Read the model definition and answer for the solid it produces. Units are mm, in the model's axes. Face numbers are marked on the shaded views. A direction names the side the tool comes from. Coordinates: 2 decimals unless noted, no trailing zeros. Order: outer loops, then holes, each group sorted by start corner. A loop starts at its lowest first (then second) coordinate and runs counter-clockwise, first axis right, second up.
from build123d import *

# Parameters (mm, degrees)
SZKIC1_W                    = 57.14
SZKIC1_H                    = 57.14
SZKIC1_R                    = 2.5
DODANIE_WYCI_GNI_CIE1_DEPTH = 5
DODANIE_WYCI_GNI_CIE2_DEPTH = 71
ZAOKR_GLENIE1_R             = 2
SZKIC3_R                    = 4
DODANIE_WYCI_GNI_CIE3_DEPTH = 20.6
ZAOKR_GLENIE2_R             = 5


with BuildPart() as part:
    # Szkic1 → Dodanie-wyciągnięcie1 (new body)
    with BuildSketch(Plane(origin=(0, 0, 0), x_dir=(1, 0, 0), z_dir=(0, 1, 0))):
        Rectangle(SZKIC1_W, SZKIC1_H)
        with Locations(Location((-23.57, 23.57, 0), (0, 0, 270))):
            Circle(SZKIC1_R, mode=Mode.SUBTRACT)
        with Locations(Location((23.57, 23.57, 0), (0, 0, 270))):
            Circle(SZKIC1_R, mode=Mode.SUBTRACT)
        with Locations(Location((23.57, -23.57, 0), (0, 0, 270))):
            Circle(SZKIC1_R, mode=Mode.SUBTRACT)
        with Locations(Location((-23.57, -23.57, 0), (0, 0, 270))):
            Circle(SZKIC1_R, mode=Mode.SUBTRACT)
    extrude(amount=DODANIE_WYCI_GNI_CIE1_DEPTH)

    # Szkic2 → Dodanie-wyciągnięcie2 (add)
    with BuildSketch(Plane(origin=(0, 5, 0), x_dir=(1, 0, 0), z_dir=(0, 1, 0))):
        with BuildLine():
            ThreePointArc((-19.07, 23.57), (-20.388019485, 20.388019485), (-23.57, 19.07))
            Line((-23.57, 19.07), (-28.57, 19.07))
            Line((-28.57, 19.07), (-28.57, -19.07))
            Line((-28.57, -19.07), (-23.57, -19.07))
            ThreePointArc((-23.57, -19.07), (-20.388019485, -20.388019485), (-19.07, -23.57))
            Line((-19.07, -23.57), (-19.07, -28.57))
            Line((-19.07, -28.57), (19.07, -28.57))
            Line((19.07, -28.57), (19.07, -23.57))
            ThreePointArc((19.07, -23.57), (20.388019485, -20.388019485), (23.57, -19.07))
            Line((23.57, -19.07), (28.57, -19.07))
            Line((28.57, -19.07), (28.57, 19.07))
            Line((28.57, 19.07), (23.57, 19.07))
            ThreePointArc((23.57, 19.07), (20.388019485, 20.388019485), (19.07, 23.57))
            Line((19.07, 23.57), (19.07, 28.57))
            Line((19.07, 28.57), (-19.07, 28.57))
            Line((-19.07, 28.57), (-19.07, 23.57))
        make_face()
    extrude(amount=DODANIE_WYCI_GNI_CIE2_DEPTH)

    # Zaokrąglenie1
    zaokr_glenie1_edges = [part.edges().sort_by_distance(p)[0] for p in [
        (19.07, 76, 26.07),
        (0, 76, 28.57),
        (-19.07, 76, 26.07),
        (-20.388019485, 76, 20.388019485),
        (-26.07, 76, 19.07),
        (-28.57, 76, 0),
        (-26.07, 76, -19.07),
        (-20.388019485, 76, -20.388019485),
        (-19.07, 76, -26.07),
        (0, 76, -28.57),
        (19.07, 76, -26.07),
        (20.388019485, 76, -20.388019485),
        (26.07, 76, -19.07),
        (28.57, 76, 0),
        (26.07, 76, 19.07),
        (20.388019485, 76, 20.388019485),
    ]]
    fillet(zaokr_glenie1_edges, radius=ZAOKR_GLENIE1_R)

    # Szkic3 → Dodanie-wyciągnięcie3 (add)
    with BuildSketch(Plane(origin=(0, 0, 0), x_dir=(-1, 0, 0), z_dir=(0, -1, 0))):
        with Locations(Location((0, 0, 0), (0, 0, 270))):
            Circle(SZKIC3_R)
    extrude(amount=DODANIE_WYCI_GNI_CIE3_DEPTH)

    # Zaokrąglenie2
    zaokr_glenie2_edges = [part.edges().sort_by_distance(p)[0] for p in [
        (-28.57, 2.5, -28.57),
        (28.57, 2.5, -28.57),
        (28.57, 2.5, 28.57),
        (-28.57, 2.5, 28.57),
    ]]
    fillet(zaokr_glenie2_edges, radius=ZAOKR_GLENIE2_R)


solid = part.part
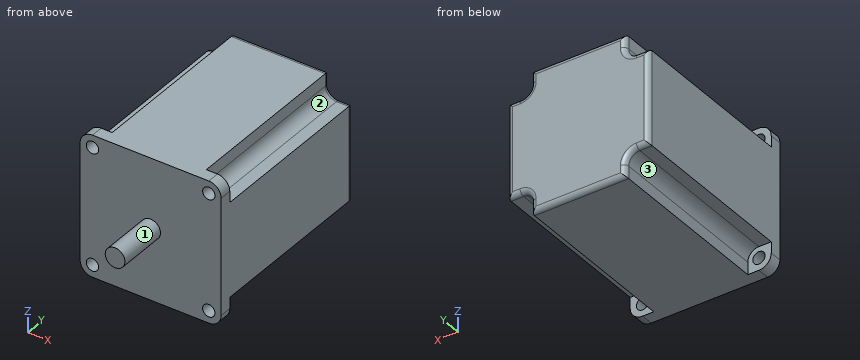
Q1. The part is cut by section C-C, the plane z = -7. Determine the outline of the cut face in (x, y), then the cut area to 3 significant figures.
Q2. Each of these flat-tipped pins is pushed along its axis until it touches: P1, Ø4, axis at y = 55, z = 26.5, coming from the -X side; P2, Ø8, axis at y = -7, z = 6, coming from the -X side; P3, Ø5.5, axis at y = 42.5, z = -25, coming from the +X side; P4, Ø4.5, axis at x = 23.57, z = -23.57, coming from the +Y side. Where does it stop, or does it pass through?
Q3. The part is cut by section D-D, the plane z = 0. Determine the outline of the cut face in (x, y).
Q4. The part is cut by section A-A, the plane y = 69. Determine the outline of the cut face in (x, z), then the cut area to 3 significant figures.
Q5. The part is cut by section B-B, the plane x = 0. Determine the outline of the cut face in (y, z), then the cut area to 3 significant figures.
Q6. Straight lines are drawn through the part: L1, parallel to X at y = 1.9, z = -23.57; L2, parallel to X at y = 1, z = -23. For each, find the intervals that lie inside material, in ascending order.
Q7. Which of the six approach directions +Z, -Z, +X, -X, +Y, -Y give full straight-line access (tool end or side, diameter ignored) to the marked faces 1, 2 and 3?
Computed values:
1. outline: (-28.57, 0) - (28.57, 0) - (28.57, 74) arc R2 ccw to (26.57, 76) - (-26.57, 76) arc R2 ccw to (-28.57, 74) - close
1. area: 4,340 mm2
2. P1: stops at x = -19.07
2. P2: stops at x = -3.46
2. P3: stops at x = 19.27
2. P4: passes through
3. outline: (-28.57, 0) - (-4, 0) - (-4, -20.6) - (4, -20.6) - (4, 0) - (28.57, 0) - (28.57, 74) arc R2 ccw to (26.57, 76) - (-26.57, 76) arc R2 ccw to (-28.57, 74) - close
4. outline: (-28.57, -19.07) - (-23.57, -19.07) arc R4.5 cw to (-19.07, -23.57) - (-19.07, -28.57) - (19.07, -28.57) - (19.07, -23.57) arc R4.5 cw to (23.57, -19.07) - (28.57, -19.07) - (28.57, 19.07) - (23.57, 19.07) arc R4.5 cw to (19.07, 23.57) - (19.07, 28.57) - (-19.07, 28.57) - (-19.07, 23.57) arc R4.5 cw to (-23.57, 19.07) - (-28.57, 19.07) - close
4. area: 2,920 mm2
5. outline: (-20.6, -4) - (0, -4) - (0, -28.57) - (74, -28.57) arc R2 ccw to (76, -26.57) - (76, 26.57) arc R2 ccw to (74, 28.57) - (0, 28.57) - (0, 4) - (-20.6, 4) - close
5. area: 4,510 mm2
6. L1: x = -28.57 to -26.07, -21.07 to 21.07, 26.07 to 28.57
6. L2: x = -28.57 to -26, -21.14 to 21.14, 26 to 28.57
7. face 1: -Y
7. face 2: +Z, +X, +Y
7. face 3: -Z, -X, +Y
